Autodesk Inventor part; units mm, degrees
ref_plane "Work Plane1" through (0, 0, 1041.4) normal (0, 0, 1) x (1, 0, 0)
ref_plane "YZ Plane" through (0, 0, 0) normal (1, 0, 0) x (0, 1, 0)
ref_plane "XZ Plane" through (0, 0, 0) normal (0, 1, 0) x (-1, 0, 0)
sketch "Sketch1" plane through (0, 0, 0) normal (0, 0, 1) x (1, 0, 0)
  line L0 (0, 0) -> (38.1, 0)
  line L1 (38.1, 76.2) -> (0, 76.2)
  line L2 (0, 76.2) -> (0, 0)
  line L3 (6.5532, 15.2924) -> (6.5532, 60.9076)
  line L4 (12.2838, 67.6723) -> (35.9776, 71.6213)
  line L5 (38.1, 76.2) -> (38.1, 74.1267)
  line L6 (12.2838, 8.5277) -> (35.9776, 4.5787)
  line L7 (38.1, 0) -> (38.1, 2.0733)
  line L8 (24.1307, 69.6468) -> (19.4329, 69.6468)
  arc A0 (38.1, 2.0733) -> (35.9776, 4.5787) centre (35.56, 2.0733) ccw
  arc A1 (35.9776, 71.6213) -> (38.1, 74.1267) centre (35.56, 74.1267) ccw
  arc A2 (6.5532, 15.2924) -> (12.2838, 8.5277) centre (13.4112, 15.2924) ccw
  arc A3 (12.2838, 67.6723) -> (6.5532, 60.9076) centre (13.4112, 60.9076) ccw
  line L9 (0, 91.44) -> (0, -15.24)
  line L10 (-7.7119, 0) -> (46.2711, 0)
  point P0 (38.1, 71.975)
  dimension "d15" = 76.2
  dimension "d25" = 6.5532
  dimension "d26" = 38.1
  dimension "d28" = 6.5532
  dimension "d29" = 2.54
  dimension "d30" = 6.858
extrude "Extrusion1" add sketch "Sketch1" along normal blind 2082.8
sketch "Sketch2" plane through (38.1, 74.1267, 2082.8) normal (1, 0, 0) x (0, 0, -1)
  line L0 (0, 0) -> (959.8939, -1.971)
  line L1 (0, -74.1267) -> (0, -4.2767)
  line L2 (0, -4.2767) -> (241.3, -74.1267)
  line L3 (241.3, -74.1267) -> (0, -74.1267)
  line L4 (2082.8, -74.1267) -> (2082.8, -4.2767)
  line L5 (2082.8, -4.2767) -> (1841.5, -74.1267)
  line L6 (1841.5, -74.1267) -> (2082.8, -74.1267)
  line L7 (2082.8, -74.1267) -> (0, -74.1267)
  line L8 (0, -74.1267) -> (0, 2.0733)
  line L9 (2082.8, 2.0733) -> (2082.8, -74.1267)
  dimension "d19" = 241.3
  dimension "d20" = 69.85
  dimension "d21" = 241.3
  dimension "d31" = 69.85
extrude "Extrusion2" cut sketch "Sketch2" against normal blind 304.8
sketch "Sketch3" plane through (6.5532, 60.9076, 2051.9082) normal (1, 0, 0) x (0, 0, -1)
  line L0 (1863.4364, -45.6153) -> (157.58, -45.6153)
  circle A0 centre (159.6082, -22.8076) radius 12.7
  line L1 (172.3082, -7.5153) -> (1848.7082, -7.5153)
  line L2 (1848.7082, -7.5153) -> (1848.7082, -42.4403)
  line L3 (1848.7082, -42.4403) -> (172.3082, -42.4403)
  line L4 (172.3082, -42.4403) -> (172.3082, -7.5153)
  line L5 (-30.8918, 8.9424) -> (-30.8918, 15.2924)
  line L6 (181.8332, -9.1028) -> (213.5832, -9.1028)
  line L7 (213.5832, -9.1028) -> (213.5832, -40.8528)
  line L8 (213.5832, -40.8528) -> (181.8332, -40.8528)
  line L9 (181.8332, -40.8528) -> (181.8332, -9.1028)
  line L10 (283.4332, -9.1028) -> (315.1832, -9.1028)
  line L11 (315.1832, -9.1028) -> (315.1832, -40.8528)
  line L12 (315.1832, -40.8528) -> (283.4332, -40.8528)
  line L13 (283.4332, -40.8528) -> (283.4332, -9.1028)
  line L14 (385.0332, -9.1028) -> (416.7832, -9.1028)
  line L15 (416.7832, -9.1028) -> (416.7832, -40.8528)
  line L16 (416.7832, -40.8528) -> (385.0332, -40.8528)
  line L17 (385.0332, -40.8528) -> (385.0332, -9.1028)
  line L18 (486.6332, -9.1028) -> (518.3832, -9.1028)
  line L19 (518.3832, -9.1028) -> (518.3832, -40.8528)
  line L20 (518.3832, -40.8528) -> (486.6332, -40.8528)
  line L21 (486.6332, -40.8528) -> (486.6332, -9.1028)
  line L22 (588.2332, -9.1028) -> (619.9832, -9.1028)
  line L23 (619.9832, -9.1028) -> (619.9832, -40.8528)
  line L24 (619.9832, -40.8528) -> (588.2332, -40.8528)
  line L25 (588.2332, -40.8528) -> (588.2332, -9.1028)
  line L26 (689.8332, -9.1028) -> (721.5832, -9.1028)
  line L27 (721.5832, -9.1028) -> (721.5832, -40.8528)
  line L28 (721.5832, -40.8528) -> (689.8332, -40.8528)
  line L29 (689.8332, -40.8528) -> (689.8332, -9.1028)
  line L30 (791.4332, -9.1028) -> (823.1832, -9.1028)
  line L31 (823.1832, -9.1028) -> (823.1832, -40.8528)
  line L32 (823.1832, -40.8528) -> (791.4332, -40.8528)
  line L33 (791.4332, -40.8528) -> (791.4332, -9.1028)
  line L34 (893.0332, -9.1028) -> (924.7832, -9.1028)
  line L35 (924.7832, -9.1028) -> (924.7832, -40.8528)
  line L36 (924.7832, -40.8528) -> (893.0332, -40.8528)
  line L37 (893.0332, -40.8528) -> (893.0332, -9.1028)
  line L38 (994.6332, -9.1028) -> (1026.3832, -9.1028)
  line L39 (1026.3832, -9.1028) -> (1026.3832, -40.8528)
  line L40 (1026.3832, -40.8528) -> (994.6332, -40.8528)
  line L41 (994.6332, -40.8528) -> (994.6332, -9.1028)
  line L42 (1096.2332, -9.1028) -> (1127.9832, -9.1028)
  line L43 (1127.9832, -9.1028) -> (1127.9832, -40.8528)
  line L44 (1127.9832, -40.8528) -> (1096.2332, -40.8528)
  line L45 (1096.2332, -40.8528) -> (1096.2332, -9.1028)
  line L46 (1197.8332, -9.1028) -> (1229.5832, -9.1028)
  line L47 (1229.5832, -9.1028) -> (1229.5832, -40.8528)
  line L48 (1229.5832, -40.8528) -> (1197.8332, -40.8528)
  line L49 (1197.8332, -40.8528) -> (1197.8332, -9.1028)
  line L50 (1299.4332, -9.1028) -> (1331.1832, -9.1028)
  line L51 (1331.1832, -9.1028) -> (1331.1832, -40.8528)
  line L52 (1331.1832, -40.8528) -> (1299.4332, -40.8528)
  line L53 (1299.4332, -40.8528) -> (1299.4332, -9.1028)
  line L54 (1401.0332, -9.1028) -> (1432.7832, -9.1028)
  line L55 (1432.7832, -9.1028) -> (1432.7832, -40.8528)
  line L56 (1432.7832, -40.8528) -> (1401.0332, -40.8528)
  line L57 (1401.0332, -40.8528) -> (1401.0332, -9.1028)
  line L58 (1502.6332, -9.1028) -> (1534.3832, -9.1028)
  line L59 (1534.3832, -9.1028) -> (1534.3832, -40.8528)
  line L60 (1534.3832, -40.8528) -> (1502.6332, -40.8528)
  line L61 (1502.6332, -40.8528) -> (1502.6332, -9.1028)
  line L62 (1604.2332, -9.1028) -> (1635.9832, -9.1028)
  line L63 (1635.9832, -9.1028) -> (1635.9832, -40.8528)
  line L64 (1635.9832, -40.8528) -> (1604.2332, -40.8528)
  line L65 (1604.2332, -40.8528) -> (1604.2332, -9.1028)
  line L66 (1705.8332, -9.1028) -> (1737.5832, -9.1028)
  line L67 (1737.5832, -9.1028) -> (1737.5832, -40.8528)
  line L68 (1737.5832, -40.8528) -> (1705.8332, -40.8528)
  line L69 (1705.8332, -40.8528) -> (1705.8332, -9.1028)
  line L70 (1807.4332, -9.1028) -> (1839.1832, -9.1028)
  line L71 (1839.1832, -9.1028) -> (1839.1832, -40.8528)
  line L72 (1839.1832, -40.8528) -> (1807.4332, -40.8528)
  line L73 (1807.4332, -40.8528) -> (1807.4332, -9.1028)
  line L74 (2051.9082, 15.2924) -> (-30.8918, 15.2924)
  line L75 (1010.5082, -7.5153) -> (1010.5082, -42.4403)
  point P0 (2051.9082, -60.9076)
  dimension "d32" = 25.4
  dimension "d33" = 34.925
  dimension "d34" = 3.175
  dimension "d35" = 1676.4
  dimension "d36" = 203.2
  dimension "d37" = 31.75
  dimension "d38" = 1.5875
  dimension "d41" = 101.6
  dimension "d46" = 190.5
  dimension "d47" = 38.1
  dimension "d48" = 9.525
  dimension "d63" = 838.2
extrude "Extrusion3" cut sketch "Sketch3" against normal blind 25.4 contours A0
hole "Hole1" at (6.5532, 38.1, 1803.4) direction (-1, 0, 0) diameter 3.5719 depth 25.4 tip angle 118
pattern_linear "Rectangular Pattern1" count 2 spacing 711.2 along (0, 0, -1) of "Hole1"
ref_plane "Work Plane1" through (0, 0, 1041.4) normal (0, 0, 1) x (1, 0, 0)
mirror "Mirror1" about plane through (0, 0, 1041.4) normal (0, 0, 1) of "Hole1", "Rectangular Pattern1"
equation "\"d21\" = d19"
equation "\"d31\" = d20"
properties part number "GE-12019-03" material "Aluminum-6061"
The listing builds one solid part. Answer for the finished solid, in the listing's coordinates (mm). Give positions to 0.01 mm unless a question says otherwise; leave off trailing zeros. Loops run counter-clockwise (first coordinate to the right, second up) from the corner with the lowest first, then second, coordinate; pieces in that order, holes last.
Item 1: Determine the mould class of faces 1 (the flat face through (6.553, 38, 1027)), 2 (the flat face through (0, 39, 1027)), 3 (the flat face through (19, 76.2, 1027)), 4 (the flat face through (5.028, 27.327, 1935.902)) for opening direction Y: +Y half, -Y half, draft (parallel to the pull), parting line (faces both ways), or undercut.
Derived:
face 1: undercut
face 2: draft
face 3: +Y half
face 4: -Y half
Item 2: A cutting plane is placed at A-A (z = 1329.5). Give the vertices of the cut face in (x, y), then the cut area to 4 significant figures.
Derived:
outline: (0, 0) - (38.1, 0) - (38.1, 2.07) arc R2.54 ccw to (35.98, 4.58) - (12.28, 8.53) arc R6.86 cw to (6.55, 15.29) - (6.55, 60.91) arc R6.86 cw to (12.28, 67.67) - (35.98, 71.62) arc R2.54 ccw to (38.1, 74.13) - (38.1, 76.2) - (0, 76.2) - close
area: 943.5 mm2
Item 3: Find the intervals of material crossed by line 1 along Y through (x, z) = (5, 990); line 2 along Y through (x, z) = (3, 1092); line 3 along X through (y, z) = (62, 1679.5), in increasing order.
Derived:
line 1: y = 0 to 36.42, 39.78 to 76.2
line 2: y = 0 to 36.33, 39.87 to 76.2
line 3: x = 0 to 6.64
Item 4: Each of these flat-tipped pins is pushed along its axis until it touches: pin 1 Ø15 at (y, z) = (38.1, 1892.3) entering from +X; pin 2 Ø5 at (y, z) = (49.5, 1289.5) entering from +X. Where does it stop, or does it pass through?
Derived:
pin 1: passes through
pin 2: stops at x = 6.55
